Part print with two shaded views. Sizes in mm from the minimum x, y, z corner. Round coordinates to 2 decimals unless told otherwise and drop trailing zeros. Write each loop counter-clockwise with the first axis right and the second up, starting at its lowest first coordinate (ties: lowest second). Pieces come first, ordered by that corner, then holes.
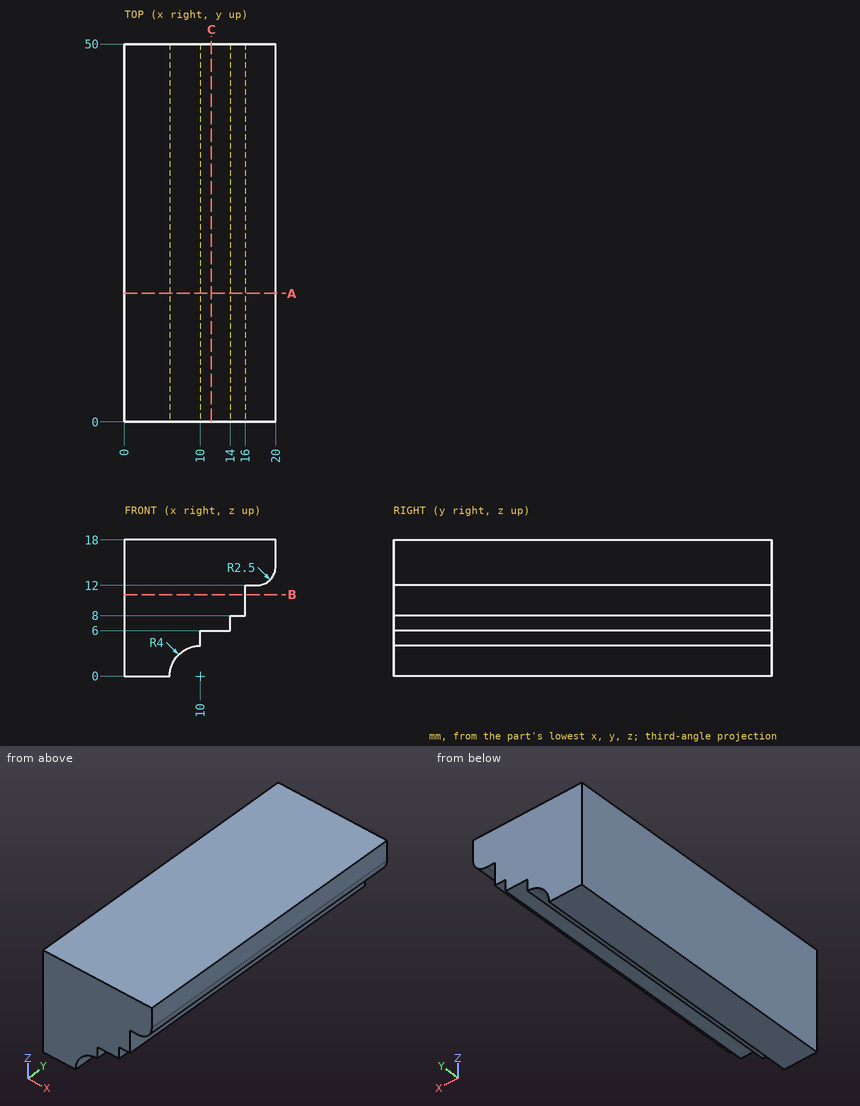
Q1. Cut at B-B on z = 10.75. Write the cut outline in (x, y).
Values follow:
outline: (0, 0) - (16, 0) - (16, 50) - (0, 50) - close
Q2. Drop flat-ended pins along their axis: pin 1 (0.6 mm diameter, centred on y = 24.5, z = 5.5, fed in from +X); pin 2 (1.6 mm diameter, centred on y = 35, z = 6.5, fed in from +X); pin 3 (2 mm diameter, centred on y = 14.5, z = 10, fed in from +X). Give the stop position or say it passes through.
Values follow:
pin 1: stops at x = 10
pin 2: stops at x = 14
pin 3: stops at x = 16
Q3. Wall check: L1, parallel to X at y = 32, z = 4.5; L2, parallel to Z at x = 14.5, y = 38; L3, parallel to X at y = 18, z = 10.25. Give the ranges that are in metal, low to high.
Values follow:
L1: x = 0 to 10
L2: z = 8 to 18
L3: x = 0 to 16
Q4. Cut at C-C on x = 11.5. Write the cut outline in (y, z).
Values follow:
outline: (0, 6) - (50, 6) - (50, 18) - (0, 18) - close
Q5. Cut at A-A on y = 17. Write the cut outline in (x, z), plus the area to 3 significant figures.
Values follow:
outline: (0, 0) - (6, 0) arc R4 cw to (10, 4) - (10, 6) - (14, 6) - (14, 8) - (16, 8) - (16, 12) - (17.5, 12) arc R2.5 ccw to (20, 14.5) - (20, 18) - (0, 18) - close
area: 258 mm2
